Could you check a few things on this model? Use its own coordinates, in mm. Face numbers are marked on the shaded views. A direction names the side the tool comes from. Give positions to 0.01 mm unless a question says otherwise; leave off trailing zeros. Loops run counter-clockwise (first coordinate to the right, second up) from the corner with the lowest first, then second, coordinate; pieces in that order, holes last. Notation, with made-up numbers: M 45,32 L 55,32 A15 cw 55,47 Z; hole C -36,-17.75 d1. An arc over 180 degrees is marked long. Answer in a Markdown table with one row per item. Add a question column.
1. I'm going to push flat-ended pins straight in: pin 1 Ø0.5 at (x, z) = (6, -32.5) entering from -Y; pin 2 Ø10 at (y, z) = (-6.5, -40.5) entering from +X; pin 3 Ø6 at (x, z) = (-1.5, -43.5) entering from +Y; pin 4 Ø1 at (y, z) = (-9, -34) entering from -X. Where does each tip first touch, or does it pass through?
2. If we section it at C-C on x = 1.25: List the corners of the cut face in (y, z) for me, then the cut area to 3 significant figures.
3. If we section it at A-A on z = -41.5: List the corners of the cut face in (x, y) for me, then the cut area to 3 significant figures.
4. I need wall thicknesses on line 1 along X through (y, z) = (-2, -41.75); line 2 along Y through (x, z) = (-3.5, -42.75); line 3 along Z through (x, y) = (8.25, 0.25). Which ranges of each line are inside material? Lowest first, please. Write a range as from..to.
5. If we section it at D-D on z = -31: List the corners of the cut face in (x, y) for me, then the cut area to 3 significant figures.
6. Which directions (+Z, -Z, +X, -X, +Y, -Y) give clear straight access to the entire face, cutting with the end or side of a thin tool? Please do the marked faces 1, 2 and 3.
7. If we section it at B-B on y = -3.75: List the corners of the cut face in (x, z) for me.
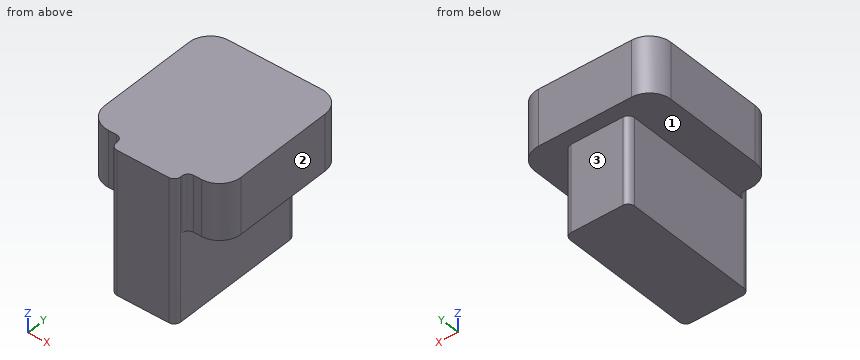
```python
from build123d import *

# Parameters (mm, degrees)
PAD001_DEPTH = 10
SKETCH003_W  = 9
SKETCH003_H  = 20
PAD002_DEPTH = 2
SKETCH004_W  = 9
SKETCH004_H  = 12.15
POCKET_DEPTH = 2
FILLET_R     = 0.9
FILLET001_R  = 3


with BuildPart() as part:
    # Sketch002 → Pad001 (new body, symmetric)
    with BuildSketch(Plane.XZ):
        Polygon((-9.5, 0), (-9.5, -7.85), (-4.5, -7.85), (-4.5, -20), (4.5, -20), (4.5, -7.85), (9.5, -7.85), (9.5, 0), align=None)
    extrude(amount=PAD001_DEPTH, both=True)

    # Sketch003 (on Face10 of Pad001) → Pad002 (join)
    with BuildSketch(Plane.XZ.offset(10)):
        with Locations((0, -10)):
            Rectangle(SKETCH003_W, SKETCH003_H)
    extrude(amount=PAD002_DEPTH)

    # Sketch004 (on Face3 of Pad002) → Pocket (cut)
    with BuildSketch(Plane(origin=(0, 10, 0), x_dir=(1, 0, 0), z_dir=(0, 1, 0))):
        with Locations((0, 13.925)):
            Rectangle(SKETCH004_W, SKETCH004_H)
    extrude(amount=-POCKET_DEPTH, mode=Mode.SUBTRACT)

    # Fillet
    fillet_edges = [part.edges().sort_by_distance(p)[0] for p in [
        (-4.5, -12, -10),
        (4.5, -12, -10),
        (4.5, 8, -13.925),
        (-4.5, 8, -13.925),
        (4.5, -10, -3.925),
        (-4.5, -10, -3.925),
    ]]
    fillet(fillet_edges, radius=FILLET_R)

    # Fillet001
    fillet001_edges = [part.edges().sort_by_distance(p)[0] for p in [
        (-9.5, -10, -3.925),
        (-9.5, 10, -3.925),
        (9.5, -10, -3.925),
        (9.5, 10, -3.925),
    ]]
    fillet(fillet001_edges, radius=FILLET001_R)


with BuildPart() as part_1:
    # Body001 placement: moved
    add(part.part.moved(Location((0, 0, -28.5))))


solid = part_1.part
```
Results:
| question | item | result |
|---|---|---|
| 1 | pin 1 | y = -10 |
| 1 | pin 2 | x = 9.5 |
| 1 | pin 3 | y = 8 |
| 1 | pin 4 | x = -9.1 |
| 2 | outline | M -12,-48.5 L 8,-48.5 L 8,-36.35 L 10,-36.35 L 10,-28.5 L -12,-28.5 Z |
| 2 | area | 416 mm2 |
| 3 | outline | M -4.5,-11.1 A0.9 ccw -3.6,-12 L 3.6,-12 A0.9 ccw 4.5,-11.1 L 4.5,7.1 A0.9 ccw 3.6,8 L -3.6,8 A0.9 ccw -4.5,7.1 Z |
| 3 | area | 179 mm2 |
| 4 | line 1 | -4.5..4.5 |
| 4 | line 2 | -12..8 |
| 4 | line 3 | -36.35..-28.5 |
| 5 | outline | M -9.5,-7 A3 ccw -6.5,-10 L -5.4,-10 A0.9 cw -4.5,-10.9 L -4.5,-11.1 A0.9 ccw -3.6,-12 L 3.6,-12 A0.9 ccw 4.5,-11.1 L 4.5,-10.9 A0.9 cw 5.4,-10 L 6.5,-10 A3 ccw 9.5,-7 L 9.5,7 A3 ccw 6.5,10 L -6.5,10 A3 ccw -9.5,7 Z |
| 5 | area | 390 mm2 |
| 6 | face 1 | -Z, +Y |
| 6 | face 2 | +Z, -Z, +X, +Y, -Y |
| 6 | face 3 | -Z, +X, -X, +Y |
| 7 | outline | M -9.5,-36.35 L -4.5,-36.35 L -4.5,-48.5 L 4.5,-48.5 L 4.5,-36.35 L 9.5,-36.35 L 9.5,-28.5 L -9.5,-28.5 Z |
